from build123d import *
from build123d.topology import SkipClean

# Parameters (mm, degrees)
SKETCH2_R           = 7.5
BOSS_EXTRUDE1_DEPTH = 18
SKETCH6_R           = 15
BOSS_EXTRUDE2_DEPTH = 18
SKETCH7_R           = 23
SKETCH7_R_2         = 15
BOSS_EXTRUDE3_DEPTH = 11
BOSS_EXTRUDE4_START = 11
SKETCH8_R           = 23
SKETCH8_R_2         = 15
BOSS_EXTRUDE4_DEPTH = 11


with BuildPart() as part:
    # Sketch2 → Boss-Extrude1 (new body)
    with BuildSketch(Plane(origin=(0, 0, 0), x_dir=(1, 0, 0), z_dir=(0, 1, 0))):
        with BuildLine():
            Line((-50.28472319, 19.35816392), (-9.579447433, 43.902799527))
            ThreePointArc((-9.579447433, 43.902799527), (11.075495329, 49.648262025), (31.730438092, 43.902799527))
            Line((31.730438092, 43.902799527), (72.435713849, 19.35816392))
            ThreePointArc((72.435713849, 19.35816392), (83.075495329, 0.518168294), (72.435713849, -18.321827333))
            Line((72.435713849, -18.321827333), (31.730438092, -42.86646294))
            ThreePointArc((31.730438092, -42.86646294), (11.075495329, -48.611925438), (-9.579447433, -42.86646294))
            Line((-9.579447433, -42.86646294), (-50.28472319, -18.321827333))
            ThreePointArc((-50.28472319, -18.321827333), (-60.924504671, 0.518168294), (-50.28472319, 19.35816392))
        make_face()
        with Locations(Location((-38.924504671, 0.518168294, 0), (0, 0, 270))):
            Circle(SKETCH2_R, mode=Mode.SUBTRACT)
        with Locations(Location((61.075495329, 0.518168294, 0), (0, 0, 270))):
            Circle(SKETCH2_R, mode=Mode.SUBTRACT)
    extrude(amount=BOSS_EXTRUDE1_DEPTH)

    # Sketch6 → Boss-Extrude2 (add)
    with BuildSketch(Plane(origin=(0, 0, 0), x_dir=(0, 0, -1), z_dir=(1, 0, 0))):
        with BuildLine():
            Line((-34.007106684, 18), (-23.507106684, 76))
            ThreePointArc((-23.507106684, 76), (-0.507106684, 99), (22.492893316, 76))
            Line((22.492893316, 76), (32.992893316, 18))
            Line((32.992893316, 18), (-34.007106684, 18))
        make_face()
        with Locations((-0.507106684, 76)):
            Circle(SKETCH6_R, mode=Mode.SUBTRACT)
    extrude(amount=BOSS_EXTRUDE2_DEPTH)

    # Sketch7 → Boss-Extrude3 (add)
    with SkipClean():  # the faces are left unmerged after this step: merging them gives an invalid solid
        with BuildSketch(Plane(origin=(18, 0, 0), x_dir=(0, 0, -1), z_dir=(1, 0, 0))):
            with Locations((-0.507106684, 76)):
                Circle(SKETCH7_R)
            with Locations((-0.507106684, 76)):
                Circle(SKETCH7_R_2, mode=Mode.SUBTRACT)
        extrude(amount=BOSS_EXTRUDE3_DEPTH)
    add(part.part.scale(1), mode=Mode.REPLACE)  # the faces are merged on a copy

    # Sketch8 → Boss-Extrude4 (add)
    with SkipClean():  # the faces are left unmerged after this step: merging them gives an invalid solid
        with BuildSketch(Plane.ZY.offset(BOSS_EXTRUDE4_START)):
            with Locations((0.507106684, 76)):
                Circle(SKETCH8_R)
            with Locations((0.507106684, 76)):
                Circle(SKETCH8_R_2, mode=Mode.SUBTRACT)
        extrude(amount=-BOSS_EXTRUDE4_DEPTH)
    add(part.part.scale(1), mode=Mode.REPLACE)  # the faces are merged on a copy


solid = part.part
CAD build for the part. Positions are in the model's coordinates, mm. A direction names the side the tool comes from. Round coordinates to 2 decimals unless told otherwise and drop trailing zeros. Write each loop counter-clockwise with the first axis right and the second up, starting at its lowest first coordinate (ties: lowest second). Pieces come first, ordered by that corner, then holes. Notation, with made-up numbers: M -37,-1 L 13,-1 A15 cw 13,16 Z; hole C 74.5,36 d4. An arc over 180 degrees is marked long. Put each result on its own line as item: value. Start each with the question number.
1) Pull direction X, two halves, no side cores. Call faces 1 (the flat face through (-29.647, 8.874, 30.766)), 2 (the cylindrical face through (-46.246, 8.874, -2.144)), 3 (the cylindrical face through (83.073, 8.874, -0.835)): pulls with the +X half, pulls with the -X half, needs draft (parallel to the pull), parting line crosses it, or undercut.
2) Saw through at A-A, the plane y = 72.5. Write the cut outline in (x, z), and give its area (3 significant figures).
3) Saw through at C-C, the plane z = 38.5. Write the cut outline in (x, y), and give its area (3 significant figures).
4) Pin check, flat tips, straight feed: pin 1 Ø4 at (y, z) = (61, 5.5) entering from -X; pin 2 Ø23 at (y, z) = (84, -0.5) entering from +X; pin 3 Ø24 at (x, z) = (61.08, -0.52) entering from +Y. Stop position of each tip, or through.
5) Saw through at B-B, the plane z = -3.5. Write the cut outline in (x, y), and give its area (3 significant figures).
6) Drill centre lines: probe 1 along Y at (x, z) = (35, 13.5); probe 2 along X at (y, z) = (65.5, -12.5). Where is each one in solid material? Low to high. Write a range as [from, to].
7) 3-axis set-ups, long thin cutter, end or side, ignore diameter. For faces 4 (the cylindrical face through (-60.922, 8.874, -0.201)), 5 (the flat face through (-11, 76, 16)), 6 (the flat face through (29, 76, -15)): which of +Z, -Z, +X, -X, +Y, -Y reach the whole face in a straight line?
8) Saw through at D-D, the plane y = 40.5. Write the cut outline in (x, z), and give its area (3 significant figures).
Resolved:
1. face 1: pulls with the -X half
1. face 2: undercut
1. face 3: pulls with the +X half
2. outline: M -11,-22.23 L 0,-22.23 L 0,-23.13 L 18,-23.13 L 18,-22.23 L 29,-22.23 L 29,-14.08 L -11,-14.08 Z; M -11,15.09 L 29,15.09 L 29,23.24 L 18,23.24 L 18,24.14 L 0,24.14 L 0,23.24 L -11,23.24 Z
2. area: 684 mm²
3. outline: M -16.82,0 L 38.97,0 L 38.97,18 L -16.82,18 Z
3. area: 1,000 mm²
4. pin 1: x = -11
4. pin 2: x = 29
4. pin 3: y = 18
5. outline: M -60.72,0 L -45.81,0 L -45.81,18 L -60.72,18 Z; M -32.04,0 L 54.19,0 L 54.19,18 L 18,18 L 18,53.35 L 29,53.35 L 29,61.55 L -11,61.55 L -11,53.35 L 0,53.35 L 0,18 L -32.04,18 Z; M -11,90.45 L 29,90.45 L 29,98.65 L -11,98.65 Z; M 67.96,0 L 82.87,0 L 82.87,18 L 67.96,18 Z
5. area: 3,380 mm²
6. probe 1: [0, 18]
6. probe 2: [-11, 29]
7. face 4: -X, +Y, -Y
7. face 5: +Z, -Z, -X, +Y
7. face 6: +Z, -Z, +X, +Y
8. outline: M 0,-28.92 L 18,-28.92 L 18,29.93 L 0,29.93 Z
8. area: 1,060 mm²
